Can you work these out from the model? Positions are in its coordinate system, mm. Give positions to 0.01 mm unless a question says otherwise; leave off trailing zeros. Write each loop counter-clockwise with the first axis right and the second up, starting at its lowest first coordinate (ties: lowest second). Pieces come first, ordered by that corner, then holes.
from build123d import *

# Parameters (mm, degrees)
SKETCH_3_R        = 6
EXTRUDE_1_DEPTH   = 4
OTHER_1_OUTLINE_R = 2
OTHER_1_DEPTH     = 4
SKETCH_14_W       = 0.1
SKETCH_14_H       = 0.08


# Read off the part's stored shape, not the designer's step: 孔1
with BuildPart() as part:
    # 草图3 → 凸台-拉伸1 (new body)
    with BuildSketch(Plane.XY):
        Circle(SKETCH_3_R)
    extrude(amount=EXTRUDE_1_DEPTH)

    # 孔1 outline → 孔1 (cut)
    with BuildSketch(Plane.XY):
        Circle(OTHER_1_OUTLINE_R)
    extrude(amount=OTHER_1_DEPTH, mode=Mode.SUBTRACT)

    # 草图11 → 切除-旋转1 (revolve, cut)
    with BuildSketch(Plane(origin=(0, 0, 0), x_dir=(0, 0, -1), z_dir=(1, 0, 0)), mode=Mode.PRIVATE) as cut_revolve_1_sk:
        Polygon((-0.3, 6), (-3.7, 6), (-2, 4.573530627), align=None)
    revolve(cut_revolve_1_sk.sketch.rotate(Axis((0, 0, 4.816901408), (0, 0, -1)), 90), axis=Axis((0, 0, 4.816901408), (0, 0, -1)), mode=Mode.SUBTRACT)

    # 草图12 → 切除-旋转2 (revolve, cut)
    with BuildSketch(Plane(origin=(0, 0, 0), x_dir=(0, 0, -1), z_dir=(1, 0, 0)), mode=Mode.PRIVATE) as cut_revolve_2_sk:
        with BuildLine():
            Line((0, 4), (-0.5, 4))
            ThreePointArc((-0.5, 4), (-0.139152669, 3.555423666), (0, 3))
            Line((0, 3), (0, 4))
        make_face()
    cut_revolve_2 = revolve(cut_revolve_2_sk.sketch.rotate(Axis((0, 0, 0), (0, 0, 1)), 90), axis=Axis((0, 0, 0), (0, 0, 1)), mode=Mode.SUBTRACT)

    # 镜向1: 切除-旋转2 across plane
    add(cut_revolve_2.mirror(Plane.XY.offset(2)), mode=Mode.SUBTRACT)

    # 草图14 → 切除-旋转3 (revolve, cut)
    with BuildSketch(Plane(origin=(0, 0, 0), x_dir=(0, 0, -1), z_dir=(1, 0, 0)), mode=Mode.PRIVATE) as cut_revolve_3_sk:
        with Locations((-0.05, 2.71)):
            Rectangle(SKETCH_14_W, SKETCH_14_H)
    cut_revolve_3 = revolve(cut_revolve_3_sk.sketch.rotate(Axis((0, 0, 0), (0, 0, 1)), 90), axis=Axis((0, 0, 0), (0, 0, 1)), mode=Mode.SUBTRACT)

    # 镜向2: 切除-旋转3 across plane
    add(cut_revolve_3.mirror(Plane.XY.offset(2)), mode=Mode.SUBTRACT)


solid = part.part
(1) Will these pins go through, and if not, where does the flat tip stop? P1, Ø2.5, axis at x = 0, y = 0, coming from the -Z side; P2, Ø2, axis at y = -3, z = 0.5, coming from the -X side.
Returned:
P1: passes through
P2: stops at x = -5.65
(2) Imagine slicing it at A-A, the plane z = 0.65. Write out the boundary of the cut face in (x, y), plus the area to 3 significant figures.
Returned:
outline: circle Ø11.41 at (0, 0); hole circle Ø4 at (0, 0)
area: 89.7 mm2
(3) If we mould it in two halves opening along X, with no side actions, what happens to faces 1 (the face through (-4.42, 4.06, 3.85)), 2 (the face through (0.867, 3.905, 0.254)), 3 (the face through (1, 2, 4))? For each: +X half, -X half, draft (parallel to the pull), parting line (faces both ways), or undercut.
Returned:
face 1: parting line
face 2: undercut
face 3: draft
(4) Imagine slicing it at B-B, the plane z = 3.05. Write out the boundary of the cut face in (x, y), plus the area to 3 significant figures.
Returned:
outline: circle Ø10.91 at (0, 0); hole circle Ø4 at (0, 0)
area: 80.9 mm2
(5) If I drill on L1, parallel to Y at x = 0, z = 0.15; L2, parallel to Z at x = 1.75, y = -5; L3, parallel to Y at x = 0, z = 1.3, over which ranges is the centre line in solid material (lowest first)?
Returned:
L1: y = -6 to -4, -3.58 to -2, 2 to 3.58, 4 to 6
L2: z = 0 to 1.14, 2.86 to 4
L3: y = -5.16 to -2, 2 to 5.16
